```python
from build123d import *

# Parameters (mm, degrees)
SM_START                          = -2
SM_BASE_FLANGE_1_OUTLINE_R        = 1.5
SM_BASE_FLANGE_1_DEPTH            = 2
SM_EDGE_FLANGE_1_STRIP_W          = 12
SM_EDGE_FLANGE_1_STRIP_H          = 2
SM_EDGE_FLANGE_1_STRIP_CUT_DEPTH  = 24
SM_EDGE_FLANGE_1_RELIEF_W         = 13
SM_EDGE_FLANGE_1_RELIEF_H         = 1
SM_EDGE_FLANGE_1_RELIEF_CUT_DEPTH = 2
SM_EDGE_FLANGE_1_DEPTH            = 24
SM_EDGE_FLANGE_1_PROFILE_W        = 24
SM_EDGE_FLANGE_1_PROFILE_H        = 10
SM_EDGE_FLANGE_1_PROFILE_R        = 1.5
SM_EDGE_FLANGE_1_FLAT_DEPTH       = 2
SM_EDGE_FLANGE_2_STRIP_W          = 12
SM_EDGE_FLANGE_2_STRIP_H          = 2
SM_EDGE_FLANGE_2_STRIP_CUT_DEPTH  = 24
SM_EDGE_FLANGE_2_RELIEF_W         = 13
SM_EDGE_FLANGE_2_RELIEF_H         = 1
SM_EDGE_FLANGE_2_RELIEF_CUT_DEPTH = 2
SM_EDGE_FLANGE_2_DEPTH            = 24
SM_EDGE_FLANGE_2_PROFILE_W        = 24
SM_EDGE_FLANGE_2_PROFILE_H        = 10
SM_EDGE_FLANGE_2_PROFILE_R        = 1.5
SM_EDGE_FLANGE_2_FLAT_DEPTH       = 2
FILLET_1_R                        = 3
CUT_EXTRUDE_1_DEPTH               = 10


# Read off the part's stored shape, not the designer's step: 基体-法兰1
# Sheet-metal steps are written as plain solids
with BuildPart() as part:
    # 基体-法兰1 outline → 基体-法兰1 (new body)
    with BuildSketch(Plane(origin=(0, 0, 0), x_dir=(1, 0, 0), z_dir=(0, 1, 0)).offset(SM_START)):
        with BuildLine():
            ThreePointArc((-50, 23), (-41.506096654, 2.493903346), (-21, -6))
            Line((-21, -6), (0, -6))
            Line((0, -6), (0, 24))
            Line((0, 24), (-20, 24))
            Line((-20, 24), (-20, 84))
            Line((-20, 84), (2, 84))
            Line((2, 84), (2, 114))
            Line((2, 114), (-21, 114))
            ThreePointArc((-21, 114), (-41.506096654, 105.506096654), (-50, 85))
            Line((-50, 85), (-50, 23))
        make_face()
        with Locations((-42.034441854, 7.71758344)):
            Circle(SM_BASE_FLANGE_1_OUTLINE_R, mode=Mode.SUBTRACT)
        with Locations((-45.727469424, 14.965558146)):
            Circle(SM_BASE_FLANGE_1_OUTLINE_R, mode=Mode.SUBTRACT)
        with Locations((-47, 23)):
            Circle(SM_BASE_FLANGE_1_OUTLINE_R, mode=Mode.SUBTRACT)
        with Locations((-36.28241656, 1.965558146)):
            Circle(SM_BASE_FLANGE_1_OUTLINE_R, mode=Mode.SUBTRACT)
        with Locations((-29.034441854, -1.727469424)):
            Circle(SM_BASE_FLANGE_1_OUTLINE_R, mode=Mode.SUBTRACT)
        with Locations((-47, 31)):
            Circle(SM_BASE_FLANGE_1_OUTLINE_R, mode=Mode.SUBTRACT)
        with Locations((-21, -3)):
            Circle(SM_BASE_FLANGE_1_OUTLINE_R, mode=Mode.SUBTRACT)
        with Locations((-21, 21)):
            Circle(SM_BASE_FLANGE_1_OUTLINE_R, mode=Mode.SUBTRACT)
        with Locations((-11, -3)):
            Circle(SM_BASE_FLANGE_1_OUTLINE_R, mode=Mode.SUBTRACT)
        with Locations((-11, 21)):
            Circle(SM_BASE_FLANGE_1_OUTLINE_R, mode=Mode.SUBTRACT)
        with Locations((-23, 31)):
            Circle(SM_BASE_FLANGE_1_OUTLINE_R, mode=Mode.SUBTRACT)
        with Locations((-47, 77)):
            Circle(SM_BASE_FLANGE_1_OUTLINE_R, mode=Mode.SUBTRACT)
        with Locations((-47, 85)):
            Circle(SM_BASE_FLANGE_1_OUTLINE_R, mode=Mode.SUBTRACT)
        with Locations((-45.727469424, 93.034441854)):
            Circle(SM_BASE_FLANGE_1_OUTLINE_R, mode=Mode.SUBTRACT)
        with Locations((-42.034441854, 100.28241656)):
            Circle(SM_BASE_FLANGE_1_OUTLINE_R, mode=Mode.SUBTRACT)
        with Locations((-36.28241656, 106.034441854)):
            Circle(SM_BASE_FLANGE_1_OUTLINE_R, mode=Mode.SUBTRACT)
        with Locations((-29.034441854, 109.727469424)):
            Circle(SM_BASE_FLANGE_1_OUTLINE_R, mode=Mode.SUBTRACT)
        with Locations((-23, 77)):
            Circle(SM_BASE_FLANGE_1_OUTLINE_R, mode=Mode.SUBTRACT)
        with Locations((-21, 87)):
            Circle(SM_BASE_FLANGE_1_OUTLINE_R, mode=Mode.SUBTRACT)
        with Locations((-14, 87)):
            Circle(SM_BASE_FLANGE_1_OUTLINE_R, mode=Mode.SUBTRACT)
        with Locations((-21, 111)):
            Circle(SM_BASE_FLANGE_1_OUTLINE_R, mode=Mode.SUBTRACT)
        with Locations((-14, 111)):
            Circle(SM_BASE_FLANGE_1_OUTLINE_R, mode=Mode.SUBTRACT)
        with Locations((-7, 87)):
            Circle(SM_BASE_FLANGE_1_OUTLINE_R, mode=Mode.SUBTRACT)
        with Locations((-7, 111)):
            Circle(SM_BASE_FLANGE_1_OUTLINE_R, mode=Mode.SUBTRACT)
    extrude(amount=SM_BASE_FLANGE_1_DEPTH)

    # 边线-法兰1 strip (across the edge) → 边线-法兰1 strip cut (cut)
    with BuildSketch(Plane(origin=(2, -2, -111), x_dir=(-1, 0, 0), z_dir=(0, 0, 1))):
        with Locations((-2, -1)):
            Rectangle(SM_EDGE_FLANGE_1_STRIP_W, SM_EDGE_FLANGE_1_STRIP_H)
    extrude(amount=SM_EDGE_FLANGE_1_STRIP_CUT_DEPTH, mode=Mode.SUBTRACT)

    # 边线-法兰1 relief (on the sheet) → 边线-法兰1 relief cut (cut)
    with BuildSketch(Plane(origin=(-2, -2, -111), x_dir=(-1, 0, 0), z_dir=(0, -1, 0))):
        with Locations((-5.5, 0.5)):
            Rectangle(SM_EDGE_FLANGE_1_RELIEF_W, SM_EDGE_FLANGE_1_RELIEF_H)
        with Locations((-5.5, -24.5)):
            Rectangle(SM_EDGE_FLANGE_1_RELIEF_W, SM_EDGE_FLANGE_1_RELIEF_H)
    extrude(amount=-SM_EDGE_FLANGE_1_RELIEF_CUT_DEPTH, mode=Mode.SUBTRACT)

    # 边线-法兰1 bend section (across the edge) → 边线-法兰1 (add)
    with BuildSketch(Plane(origin=(2, -2, -111), x_dir=(-1, 0, 0), z_dir=(0, 0, 1))):
        with BuildLine():
            Line((0, 2), (2, 2))
            ThreePointArc((2, 2), (2.585786438, 0.585786438), (4, 0))
            Line((4, 0), (4, -2))
            ThreePointArc((4, -2), (1.171572875, -0.828427125), (0, 2))
        make_face()
    extrude(amount=SM_EDGE_FLANGE_1_DEPTH)

    # 边线-法兰1 profile (on flange) → 边线-法兰1 flat (add)
    with BuildSketch(Plane(origin=(2, -2, 0), x_dir=(0, 0, 1), z_dir=(1, 0, 0))):
        with Locations((-99, 7)):
            Rectangle(SM_EDGE_FLANGE_1_PROFILE_W, SM_EDGE_FLANGE_1_PROFILE_H)
        with Locations((-91, 7)):
            Circle(SM_EDGE_FLANGE_1_PROFILE_R, mode=Mode.SUBTRACT)
        with Locations((-107, 7)):
            Circle(SM_EDGE_FLANGE_1_PROFILE_R, mode=Mode.SUBTRACT)
    extrude(amount=-SM_EDGE_FLANGE_1_FLAT_DEPTH)

    # 边线-法兰2 strip (across the edge) → 边线-法兰2 strip cut (cut)
    with BuildSketch(Plane(origin=(0, -2, -21), x_dir=(-1, 0, 0), z_dir=(0, 0, 1))):
        with Locations((-2, -1)):
            Rectangle(SM_EDGE_FLANGE_2_STRIP_W, SM_EDGE_FLANGE_2_STRIP_H)
    extrude(amount=SM_EDGE_FLANGE_2_STRIP_CUT_DEPTH, mode=Mode.SUBTRACT)

    # 边线-法兰2 relief (on the sheet) → 边线-法兰2 relief cut (cut)
    with BuildSketch(Plane(origin=(-4, -2, -21), x_dir=(-1, 0, 0), z_dir=(0, -1, 0))):
        with Locations((-5.5, 0.5)):
            Rectangle(SM_EDGE_FLANGE_2_RELIEF_W, SM_EDGE_FLANGE_2_RELIEF_H)
        with Locations((-5.5, -24.5)):
            Rectangle(SM_EDGE_FLANGE_2_RELIEF_W, SM_EDGE_FLANGE_2_RELIEF_H)
    extrude(amount=-SM_EDGE_FLANGE_2_RELIEF_CUT_DEPTH, mode=Mode.SUBTRACT)

    # 边线-法兰2 bend section (across the edge) → 边线-法兰2 (add)
    with BuildSketch(Plane(origin=(0, -2, -21), x_dir=(-1, 0, 0), z_dir=(0, 0, 1))):
        with BuildLine():
            Line((0, 2), (2, 2))
            ThreePointArc((2, 2), (2.585786438, 0.585786438), (4, 0))
            Line((4, 0), (4, -2))
            ThreePointArc((4, -2), (1.171572875, -0.828427125), (0, 2))
        make_face()
    extrude(amount=SM_EDGE_FLANGE_2_DEPTH)

    # 边线-法兰2 profile (on flange) → 边线-法兰2 flat (add)
    with BuildSketch(Plane(origin=(0, -2, 0), x_dir=(0, 0, 1), z_dir=(1, 0, 0))):
        with Locations((-9, 7)):
            Rectangle(SM_EDGE_FLANGE_2_PROFILE_W, SM_EDGE_FLANGE_2_PROFILE_H)
        with Locations((-1, 7)):
            Circle(SM_EDGE_FLANGE_2_PROFILE_R, mode=Mode.SUBTRACT)
        with Locations((-17, 7)):
            Circle(SM_EDGE_FLANGE_2_PROFILE_R, mode=Mode.SUBTRACT)
    extrude(amount=-SM_EDGE_FLANGE_2_FLAT_DEPTH)

    # 圆角1
    fillet_1_edges = [part.edges().sort_by_distance(p)[0] for p in [
        (1, -14, -111),
        (1, -14, -87),
        (-1, -14, -21),
        (-1, -14, 3),
    ]]
    fillet(fillet_1_edges, radius=FILLET_1_R)

    # 草图13 → 切除-拉伸1 (cut)
    with BuildSketch(Plane(origin=(0, 0, 0), x_dir=(1, 0, 0), z_dir=(0, 1, 0))):
        with BuildLine():
            Line((-37, 77), (-37, 58))
            ThreePointArc((-37, 58), (-39, 56), (-41, 58))
            Line((-41, 58), (-41, 77))
            ThreePointArc((-41, 77), (-39, 79), (-37, 77))
        make_face()
        with BuildLine():
            Line((-29, 77), (-29, 58))
            ThreePointArc((-29, 58), (-31, 56), (-33, 58))
            Line((-33, 58), (-33, 77))
            ThreePointArc((-33, 77), (-31, 79), (-29, 77))
        make_face()
        with BuildLine():
            Line((-29, 31), (-29, 50))
            ThreePointArc((-29, 50), (-31, 52), (-33, 50))
            Line((-33, 50), (-33, 31))
            ThreePointArc((-33, 31), (-31, 29), (-29, 31))
        make_face()
        with BuildLine():
            Line((-37, 31), (-37, 50))
            ThreePointArc((-37, 50), (-39, 52), (-41, 50))
            Line((-41, 50), (-41, 31))
            ThreePointArc((-41, 31), (-39, 29), (-37, 31))
        make_face()
        with BuildLine():
            Line((-14, 105), (-7, 105))
            ThreePointArc((-7, 105), (-5, 103), (-7, 101))
            Line((-7, 101), (-14, 101))
            ThreePointArc((-14, 101), (-16, 103), (-14, 105))
        make_face()
        with BuildLine():
            Line((-14, 93), (-7, 93))
            ThreePointArc((-7, 93), (-5, 95), (-7, 97))
            Line((-7, 97), (-14, 97))
            ThreePointArc((-14, 97), (-16, 95), (-14, 93))
        make_face()
        with BuildLine():
            Line((-14, 3), (-7, 3))
            ThreePointArc((-7, 3), (-5, 5), (-7, 7))
            Line((-7, 7), (-14, 7))
            ThreePointArc((-14, 7), (-16, 5), (-14, 3))
        make_face()
        with BuildLine():
            Line((-14, 15), (-7, 15))
            ThreePointArc((-7, 15), (-5, 13), (-7, 11))
            Line((-7, 11), (-14, 11))
            ThreePointArc((-14, 11), (-16, 13), (-14, 15))
        make_face()
        with BuildLine():
            ThreePointArc((-21, 105), (-35.142135624, 99.142135624), (-41, 85))
            ThreePointArc((-41, 85), (-39, 83), (-37, 85))
            ThreePointArc((-37, 85), (-32.313708499, 96.313708499), (-21, 101))
            ThreePointArc((-21, 101), (-19, 103), (-21, 105))
        make_face()
        with BuildLine():
            ThreePointArc((-21, 97), (-29.485281374, 93.485281374), (-33, 85))
            ThreePointArc((-33, 85), (-31, 83), (-29, 85))
            ThreePointArc((-29, 85), (-26.656854249, 90.656854249), (-21, 93))
            ThreePointArc((-21, 93), (-19, 95), (-21, 97))
        make_face()
        with BuildLine():
            ThreePointArc((-21, 3), (-35.142135624, 8.857864376), (-41, 23))
            ThreePointArc((-41, 23), (-39, 25), (-37, 23))
            ThreePointArc((-37, 23), (-32.313708499, 11.686291501), (-21, 7))
            ThreePointArc((-21, 7), (-19, 5), (-21, 3))
        make_face()
        with BuildLine():
            ThreePointArc((-21, 11), (-29.485281374, 14.514718626), (-33, 23))
            ThreePointArc((-33, 23), (-31, 25), (-29, 23))
            ThreePointArc((-29, 23), (-26.656854249, 17.343145751), (-21, 15))
            ThreePointArc((-21, 15), (-19, 13), (-21, 11))
        make_face()
    extrude(amount=-CUT_EXTRUDE_1_DEPTH, mode=Mode.SUBTRACT)


solid = part.part
```
Input: part model. Units: mm. Frame: model coordinates. A direction names the side the tool comes from. Coordinates: 2 decimals unless noted, no trailing zeros. Loops run counter-clockwise (first coordinate to the right, second up) from the corner with the lowest first, then second, coordinate; pieces in that order, holes last. Notation, with made-up numbers: (66, 42.5) -> (120, 42.5) arc R32 ccw to (120, 68.5) -> close; hole circle Ø4 at (24.25, 11). An arc over 180 degrees is marked (long way). Use a Markdown table: item, result.
1) Material intervals for line 1 along Z through (x, y) = (-0.9, -9); line 2 along X through (y, z) = (-1.75, -4.5); line 3 along Z through (x, y) = (-18.5, -1), sorted ascending. Write a range as from..to.
Results found:
| item | result |
|---|---|
| line 1 | z = -21..-18.5, -15.5..-2.5, 0.5..3 |
| line 2 | x = -43.33..-28.6, -19.06..-15.94, -5.06..-0.69 |
| line 3 | z = -114..-84, -24..6 |
2) Pull-direction query (X, two-part tool) for faces 1 (the flat face through (-50, -1, -54)), 2 (the cylindrical face through (-22.11, -1.01, -22.01)), 3 (the flat face through (-30, -2, -55)); classes: released by +X, released by -X, zero draft, split by the parting line, or undercut.
Results found:
| item | result |
|---|---|
| face 1 | released by -X |
| face 2 | undercut |
| face 3 | zero draft |
3) Cut plane B-B (z = -36). Return the cut outline in (x, y).
Results found:
| item | result |
|---|---|
| outline | (-50, -2) -> (-41, -2) -> (-41, 0) -> (-50, 0) -> close; (-37, -2) -> (-33, -2) -> (-33, 0) -> (-37, 0) -> close; (-29, -2) -> (-20, -2) -> (-20, 0) -> (-29, 0) -> close |
4) Contact query for flat-ended pins moving along their axis: pin 1 (1.6 mm diameter, centred on y = -1.5, z = -40, fed in from +X); pin 2 (2 mm diameter, centred on x = -42.5, z = -20, fed in from -Y); pin 3 (5 mm diameter, centred on y = -8.5, z = -8, fed in from +X). Output: stop coordinate, or through.
Results found:
| item | result |
|---|---|
| pin 1 | stops at x = -20 |
| pin 2 | stops at y = -2 |
| pin 3 | stops at x = 0 |
5) Cut plane A-A (x = -11). Give the number of separate pieces and of enclosed holes in the cut face, then the cut area to 3 significant figures.
Results found:
| item | result |
|---|---|
| separate pieces | 8 |
| enclosed holes | 0 |
| area | 76.0 mm2 |
6) Access query for faces 4 (the cylindrical face through (-39, -1, -56)), 5 (the flat face through (-2, -9, -9)), 6 (the flat face through (2, -1, -85)). Directions: +Z, -Z, +X, -X, +Y, -Y. A direction counts if a zero-diameter tool reaches every point of the face in a straight line with its end or side. Return the directions, or none.
Results found:
| item | result |
|---|---|
| face 4 | +Y, -Y |
| face 5 | +Z, -Z, -X, -Y |
| face 6 | +Z, -Z, +X, +Y, -Y |
